```python
from build123d import *

# Parameters (mm, degrees)
SCHNITT_LINEAR_AUSTRAGEN3_REACH = 10
SKIZZE3_R                       = 1
SCHNITT_LINEAR_AUSTRAGEN4_REACH = 10
SKIZZE3_4_R                     = 11
SKIZZE3_4_R_2                   = 1.5
SCHNITT_LINEAR_AUSTRAGEN5_DEPTH = 5
SCHNITT_LINEAR_AUSTRAGEN6_REACH = 10
SKIZZE3_5_R                     = 1.5


with BuildPart() as part:
    # Skizze1 → Rotation2 (revolve)
    with BuildSketch(Plane(origin=(0, 0, 0), x_dir=(0, 0, -1), z_dir=(1, 0, 0))):
        with BuildLine():
            Line((0.380209453, 2.098852641), (30.229832566, 2.098852641))
            add(Edge.make_bspline(
                [(29.260449341, 10.098852641), (29.33429968, 7.417548621), (29.681552607, 4.815540148), (30.229832566, 2.098852641)],
                knots=[0.538089657, 0.538089657, 0.538089657, 0.538089657, 1, 1, 1, 1], degree=3))
            Line((29.260449341, 10.098852641), (0.380209453, 10.098852641))
            Line((0.380209453, 10.098852641), (0.380209453, 5.098852641))
            Line((0.380209453, 5.098852641), (0.380209453, 2.098852641))
        make_face()
    revolve(axis=Axis((0, 5.098852641, -0.380209453), (0, 1, 0)))

    # Skizze3 → Schnitt-Linear austragen3 (cut, up to next)
    with BuildSketch(Plane(origin=(0, 10.098852641, 0), x_dir=(1, 0, 0), z_dir=(0, 1, 0)), mode=Mode.PRIVATE) as schnitt_linear_austragen3_sk1:
        with Locations((0, -20)):
            Circle(SKIZZE3_R)
    schnitt_linear_austragen3_tool1 = extrude(schnitt_linear_austragen3_sk1.sketch, amount=-SCHNITT_LINEAR_AUSTRAGEN3_REACH, mode=Mode.PRIVATE) & part.part
    add(schnitt_linear_austragen3_tool1.solids().sort_by_distance((0, 10.098853, 20))[0], mode=Mode.SUBTRACT)
    # Skizze3 → Schnitt-Linear austragen3 (cut, up to next)
    with BuildSketch(Plane(origin=(0, 10.098852641, 0), x_dir=(1, 0, 0), z_dir=(0, 1, 0)), mode=Mode.PRIVATE) as schnitt_linear_austragen3_sk2:
        with Locations((0, 20)):
            Circle(SKIZZE3_R)
    schnitt_linear_austragen3_tool2 = extrude(schnitt_linear_austragen3_sk2.sketch, amount=-SCHNITT_LINEAR_AUSTRAGEN3_REACH, mode=Mode.PRIVATE) & part.part
    add(schnitt_linear_austragen3_tool2.solids().sort_by_distance((0, 10.098853, -20))[0], mode=Mode.SUBTRACT)

    # Skizze3_3 → Schnitt-Linear austragen4 (cut, up to next)
    with BuildSketch(Plane(origin=(0, 10.098852641, 0), x_dir=(1, 0, 0), z_dir=(0, 1, 0)), mode=Mode.PRIVATE) as schnitt_linear_austragen4_sk1:
        with BuildLine():
            ThreePointArc((-8.113636364, -1.493788793), (0.75, -8.215838363), (8.25, 0))
            ThreePointArc((8.25, 0), (0.75, 8.215838363), (-8.113636364, 1.493788793))
            ThreePointArc((-8.113636364, 1.493788793), (-7.142176581, 1.011299794), (-6.75, 0))
            ThreePointArc((-6.75, 0), (-7.142176581, -1.011299794), (-8.113636364, -1.493788793))
        make_face()
    schnitt_linear_austragen4_tool1 = extrude(schnitt_linear_austragen4_sk1.sketch, amount=-SCHNITT_LINEAR_AUSTRAGEN4_REACH, mode=Mode.PRIVATE) & part.part
    add(schnitt_linear_austragen4_tool1.solids().sort_by_distance((0.122549, 10.098853, 0))[0], mode=Mode.SUBTRACT)

    # Skizze3_4 → Schnitt-Linear austragen5 (cut)
    with BuildSketch(Plane(origin=(0, 10.098852641, 0), x_dir=(1, 0, 0), z_dir=(0, 1, 0))):
        Circle(SKIZZE3_4_R)
        with Locations((-8.25, 0)):
            Circle(SKIZZE3_4_R_2, mode=Mode.SUBTRACT)
    extrude(amount=-SCHNITT_LINEAR_AUSTRAGEN5_DEPTH, mode=Mode.SUBTRACT)

    # Skizze3_5 → Schnitt-Linear austragen6 (cut, up to next)
    with BuildSketch(Plane(origin=(0, 10.098852641, 0), x_dir=(1, 0, 0), z_dir=(0, 1, 0)), mode=Mode.PRIVATE) as schnitt_linear_austragen6_sk1:
        with Locations((-8.25, 0)):
            Circle(SKIZZE3_5_R)
    schnitt_linear_austragen6_tool1 = extrude(schnitt_linear_austragen6_sk1.sketch, amount=-SCHNITT_LINEAR_AUSTRAGEN6_REACH, mode=Mode.PRIVATE) & part.part
    add(schnitt_linear_austragen6_tool1.solids().sort_by_distance((-8.25, 10.098853, 0))[0], mode=Mode.SUBTRACT)


solid = part.part
```
CAD build for the part. Positions are in the model's coordinates, mm. A direction names the side the tool comes from. Coordinates: 2 decimals unless noted, no trailing zeros. Return JSON: item names as keys, results as strings. Group by question number.
Q1. Drill centre lines: line 1 (Z direction, x = 0, y = 7.9); line 2 (Z direction, x = 0, y = 6); line 3 (Z direction, x = -7, y = 5.5). Where is each one in solid material? Low to high.
Q2. Cut at A-A, the plane y = 3. State how many separate pieces and enclosed holes the cut face has, then the cut area to 3 significant figures.
Q3. Pull direction Z, two halves, no side cores. Call faces 3 (the face through (0, 10.099, -13)), 4 (the face through (-2.38, 7.63, 10.74)), 5 (the face through (2.4, 5.099, 8.1)): released by +Z, released by -Z, zero draft, split by the parting line, or undercut.
Q4. Which spindle directions (+Z, -Z, +X, -X, +Y, -Y) get a long thin tool onto all of the face, cutting with end or side? Do faces 1 (the face through (6, 2.099, 6)), 2 (the face through (-9.75, 3.62, -0.03)). Say none if no direction does.
Q5. Flat gauge pins, fed straight in: pin 1 (3.5 mm diameter, centred on x = -8.25, z = 0, fed in from +Y); pin 2 (3 mm diameter, centred on x = -12.5, y = 6.5, fed in from -Z); pin 3 (1.5 mm diameter, centred on x = 23, y = 5, fed in from +Z). Where does each tip first touch, or does it go through?
Returned:
{
 "1": {"line 1": "z = -29.38 to -21, -19 to -11, 11 to 19, 21 to 28.62", "line 2": "z = -29.58 to -21, -19 to -11, 11 to 19, 21 to 28.82", "line 3": "z = -28.8 to -8.49, 8.49 to 28.04"},
 "2": {"separate pieces": "1", "enclosed holes": "3", "area": "2,540 mm2"},
 "3": {"face 3": "zero draft", "face 4": "undercut", "face 5": "undercut"},
 "4": {"face 1": "+Z, -Z, +X, -X, -Y", "face 2": "+Y, -Y"},
 "5": {"pin 1": "stops at y = 5.1", "pin 2": "stops at z = -27.4", "pin 3": "stops at z = 18.76"}
}
